Work out the finished part from the listing and answer in its coordinate system (mm). Face numbers are marked on the shaded views. Coordinates: 2 decimals unless noted, no trailing zeros. Order: outer loops, then holes, each group sorted by start corner. A loop starts at its lowest first (then second) coordinate and runs counter-clockwise, first axis right, second up. Notation, with made-up numbers: M 20.5,28 L 74.5,28 A27 cw 74.5,53 Z; hole C -1.75,81 d5. An arc over 180 degrees is marked long. Answer in a Markdown table with one row per item. Add a question column.
Item 1: The part is cut by section D-D (y = 12). Write down the section's boundary in (x, z), then the cut area to 3 significant figures.
Item 2: The mould has two halves that part along X. Classify the marked faces 1, 2 and 3: released by +X, released by -X, zero draft, split by the parting line, or undercut.
Item 3: The part is cut by section C-C (z = 34.5). Write down the section's boundary in (x, y), then the cut area to 3 significant figures.
Item 4: Flat-ended cylindrical pins translate along their axes: pin 1 Ø1.1 at (x, z) = (16, -36) entering from +Y; pin 2 Ø0.6 at (x, z) = (16, 0) entering from +Y; pin 3 Ø5 at (x, y) = (10.5, 8) entering from -Z; pin 4 Ø12.5 at (x, z) = (-1, -1.5) entering from +Y. Find the tip coordinate at first contact, or state that the pin passes through.
Item 5: Consider line 1 (X direction, y = 6.75, z = -32.5); line 2 (X direction, y = 8.15, z = 0); line 3 (X direction, y = 2.7, z = 0). Determine where each line is inside the solid, lowest interval first. Write a range as from..to.
Item 6: The part is cut by section B-B (x = 0). Write down the section's boundary in (y, z), then the cut area to 3 significant figures.
Item 7: The part is cut by section A-A (y = 2.25). Write down the section's boundary in (x, z).
Autodesk Inventor part; units mm, degrees
ref_plane "YZ Plane" through (0, 0, 0) normal (1, 0, 0) x (0, 1, 0)
ref_plane "XZ Plane" through (0, 0, 0) normal (0, 1, 0) x (-1, 0, 0)
ref_plane "XY Plane" through (0, 0, 0) normal (0, 0, 1) x (1, 0, 0)
sketch "Sketch1" plane through (0, 0, 0) normal (0, 1, 0) x (-1, 0, 0)
  circle A0 centre (0, 0) radius 13.8
  circle A1 centre (0, 0) radius 5
  circle A2 centre (0, 0) radius 6
  dimension "d0" = 27.6
  dimension "d1" = 10
  dimension "d2" = 12
extrude "Extrusion1" add sketch "Sketch1" along normal blind 5 contours A0
sketch "Sketch2" plane through (0, 0, 0) normal (0, -1, 0) x (1, 0, 0)
  circle A0 centre (0, 0) radius 6
  line L0 (6, 0) -> (13.8, 0)
  circle A1 centre (0, 0) radius 13.8
  line L1 (13.8, -40) -> (6, -40)
  line L2 (6, -40) -> (6, 40)
  line L3 (6, 40) -> (13.8, 40)
  line L4 (13.8, 40) -> (13.8, -40)
  line L5 (13.8, -40) -> (6, 40) construction
  line L6 (6, -40) -> (13.8, 40) construction
  line L7 (17.7, 40) -> (9.9, 40)
  line L8 (9.9, 40) -> (9.9, -40)
  line L9 (9.9, -40) -> (17.7, -40)
  line L10 (17.7, -40) -> (17.7, 40)
  line L11 (17.7, 40) -> (9.9, -40) construction
  line L12 (9.9, 40) -> (17.7, -40) construction
  point P0 (9.9, 0)
  point P1 (6, -12.4274)
  point P2 (6, 12.4274)
  dimension "d5" = 80
extrude "Extrusion2" add sketch "Sketch2" against normal blind 5 contours A1 L8 L1 L2 | L2 L3 L8 A1 | L4 L1 L8 A1 | A1 L8 L3 L4 | L4 L7 L10 L9
sketch "Sketch3" plane through (6, 0, 40) normal (0, 0, 1) x (1, 0, 0)
  line L0 (-12, 5) -> (0, 5)
  line L1 (7.8, 0) -> (0, 0)
  line L2 (0, 5) -> (7.8, 0) construction
  line L3 (0, 5) -> (7.8, 5) construction
  line L4 (0, 0) -> (7.8, 5) construction
  point P0 (-6, 0)
sketch "Sketch4" plane through (6, 0, 40) normal (0, 0, 1) x (1, 0, 0)
  line L0 (0, 0) -> (0, 5)
  line L1 (0, 2.5) -> (11.7, 2.5)
  line L2 (11.7, 0) -> (11.7, 5)
  line L3 (5.85, 2.5) -> (5.85, 5)
  line L4 (0, 5) -> (11.7, 5)
  circle A0 centre (5.85, 5) radius 3.5
  point P0 (-6, 0)
  point P1 (2.35, 5)
  point P2 (9.35, 5)
  dimension "d8" = 7
extrude "Extrusion3" cut sketch "Sketch4" against normal through all contours A0 L4 L3 L1 | L1 A0 | L3 L4 A0 L1
sketch "Sketch5" plane through (0, 5, 0) normal (0, 1, 0) x (1, 0, 0)
  line L0 (17.7, -40) -> (6, -40)
  line L1 (8.35, -40) -> (8.35, 40)
  line L2 (6, -40) -> (8.35, -40)
  line L3 (8.35, -40) -> (8.35, -31)
  line L4 (8.35, -31) -> (6, -31)
  line L5 (6, -31) -> (6, -40)
  line L6 (15.35, 40) -> (15.35, -40)
  line L7 (17.7, -40) -> (17.7, 40)
  line L8 (15.35, -40) -> (17.7, -40)
  line L9 (17.7, -40) -> (17.7, -31)
  line L10 (17.7, -31) -> (15.35, -31)
  line L11 (15.35, -31) -> (15.35, -40)
  point P0 (0, 0)
  dimension "d11" = 9
extrude "Extrusion4" add sketch "Sketch5" along normal blind 10 contours L0 L5 L4 L1
extrude "Extrusion5" add sketch "Sketch5" along normal blind 5 contours L0 L6 L10 L7
mirror "Mirror1" about plane through (0, 0, 0) normal (0, 0, 1) of "Extrusion4", "Extrusion5"
sketch "Sketch6" plane through (0, 5, 0) normal (0, 1, 0) x (1, 0, 0)
  circle A0 centre (0, 0) radius 8.35
  circle A1 centre (0, 0) radius 6
extrude "Extrusion6" add sketch "Sketch6" along normal blind 6
chamfer "Chamfer1" distance 0.5 angle 45 14 edges at (-8.35, 11, 0) (-6, 11, 0) (-13.8, 5, 0) (6, 5, -21.7137) (6, 5, 21.7137) (8.35, 15, 35.5) (6, 15, 35.5) (8.35, 15, -35.5) (6, 15, -35.5) (17.7, 10, -35.5) (15.35, 10, -35.5) (17.7, 10, 35.5) (15.35, 10, 35.5) (17.7, 5, 0)
properties part number "ipad holder"
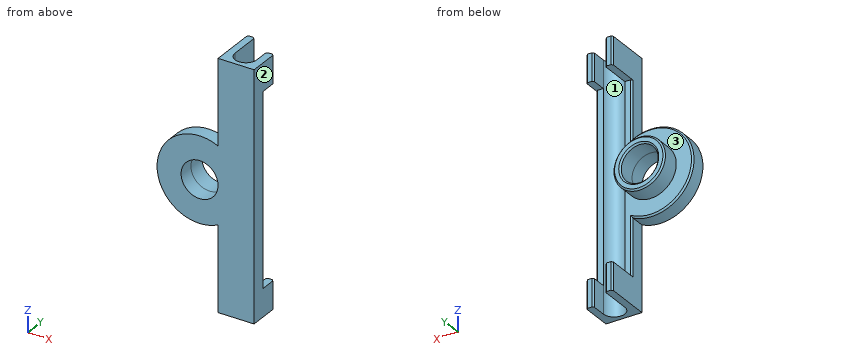
Reply:
| question | item | result |
|---|---|---|
| 1 | outline | M 6,-40 L 8.35,-40 L 8.35,-31 L 6,-31 Z; M 6,31 L 8.35,31 L 8.35,40 L 6,40 Z |
| 1 | area | 42.3 mm2 |
| 2 | face 1 | undercut |
| 2 | face 2 | released by +X |
| 2 | face 3 | zero draft |
| 3 | outline | M 6,0 L 17.7,0 L 17.7,9.5 L 17.2,10 L 15.85,10 L 15.35,9.5 L 15.35,5 A3.5 cw 8.35,5 L 8.35,14.5 L 7.85,15 L 6.5,15 L 6,14.5 Z |
| 3 | area | 74.0 mm2 |
| 4 | pin 1 | stops at y = 10 |
| 4 | pin 2 | stops at y = 5 |
| 4 | pin 3 | stops at z = -40 |
| 4 | pin 4 | stops at y = 11 |
| 5 | line 1 | x = 6..8.35, 15.35..17.7 |
| 5 | line 2 | x = -8.35..-6, 6..8.35 |
| 5 | line 3 | x = -13.8..-6, 6..9.21, 14.49..17.7 |
| 6 | outline | M 0,-13.8 L 4.5,-13.8 L 5,-13.3 L 5,-8.35 L 10.5,-8.35 L 11,-7.85 L 11,-6.5 L 10.5,-6 L 0,-6 Z; M 0,6 L 10.5,6 L 11,6.5 L 11,7.85 L 10.5,8.35 L 5,8.35 L 5,13.3 L 4.5,13.8 L 0,13.8 Z |
| 6 | area | 105 mm2 |
| 7 | outline | M 6,-40 L 9.68,-40 L 9.68,40 L 6,40 L 6,12.43 A13.8 ccw long 6,-12.43 Z; M 14.02,-40 L 17.7,-40 L 17.7,40 L 14.02,40 Z; hole C 0,0 d12 |
